Verification items for the finished model (mm, model axes). Round coordinates to 2 decimals unless told otherwise and drop trailing zeros. Order: outer loops, then holes, each group sorted by start corner. A loop starts at its lowest first (then second) coordinate and runs counter-clockwise, first axis right, second up. Notation, with made-up numbers: (-9, 3.25) -> (11, 3.25) arc R17 cw to (11, 25.25) -> close; hole circle Ø2 at (51, 74.5). An arc over 180 degrees is marked (long way). Write item = value, one per line. Start each with the question number.
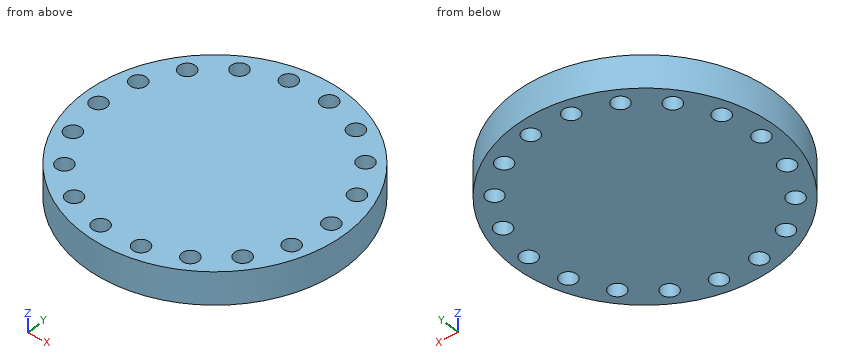
from build123d import *

# Parameters (mm, degrees)
SKETCH1_R           = 50.8
BOSS_EXTRUDE2_DEPTH = 12.7
SKETCH1_7_R         = 3.175
CUT_EXTRUDE1_DEPTH  = 12.7


with BuildPart() as part:
    # Sketch1 → Boss-Extrude2 (new body)
    with BuildSketch(Plane.XY):
        Circle(SKETCH1_R)
    extrude(amount=-BOSS_EXTRUDE2_DEPTH)

    # Sketch1<7> → Cut-Extrude1 (cut)
    with BuildSketch(Plane.XY):
        with Locations((-44.45, 0)):
            Circle(SKETCH1_7_R)
        with Locations((-41.769336994, 15.202795371)):
            Circle(SKETCH1_7_R)
        with Locations((-34.050675497, 28.571909251)):
            Circle(SKETCH1_7_R)
        with Locations((-22.225, 38.494829198)):
            Circle(SKETCH1_7_R)
        with Locations((-7.718661497, 43.774704621)):
            Circle(SKETCH1_7_R)
        with Locations((7.718661497, 43.774704621)):
            Circle(SKETCH1_7_R)
        with Locations((22.225, 38.494829198)):
            Circle(SKETCH1_7_R)
        with Locations((34.050675497, 28.571909251)):
            Circle(SKETCH1_7_R)
        with Locations((41.769336994, 15.202795371)):
            Circle(SKETCH1_7_R)
        with Locations((44.45, 0)):
            Circle(SKETCH1_7_R)
        with Locations((41.769336994, -15.202795371)):
            Circle(SKETCH1_7_R)
        with Locations((34.050675497, -28.571909251)):
            Circle(SKETCH1_7_R)
        with Locations((22.225, -38.494829198)):
            Circle(SKETCH1_7_R)
        with Locations((7.718661497, -43.774704621)):
            Circle(SKETCH1_7_R)
        with Locations((-7.718661497, -43.774704621)):
            Circle(SKETCH1_7_R)
        with Locations((-22.225, -38.494829198)):
            Circle(SKETCH1_7_R)
        with Locations((-34.050675497, -28.571909251)):
            Circle(SKETCH1_7_R)
        with Locations((-41.769336994, -15.202795371)):
            Circle(SKETCH1_7_R)
    extrude(amount=-CUT_EXTRUDE1_DEPTH, mode=Mode.SUBTRACT)


solid = part.part
(1) Cross-section at B-B (x = -35.5). Enter the section's corners in (y, z), and give its area (3 significant figures).
(2) Cross-section at D-D (y = 22). Enter the section's corners in (x, z).
(3) Depth check by flat-ended pin: pin 1 (4 mm diameter, centred on x = 34.05, y = 28.57, fed in from -Z); pin 2 (7.5 mm diameter, centred on x = 41.77, y = -15.2, fed in from -Z); pin 3 (3 mm diameter, centred on y = -4.5, z = -11.5, fed in from -X); pin 4 (5 mm diameter, centred on y = -3.5, z = -10.5, fed in from +X). Enter the tip coordinate at first touch or a pass-through.
(4) Scan lines: line 1 along X through (y, z) = (-31, -0.75); line 2 along X through (y, z) = (-40, -11); line 3 along Y through (x, z) = (-6.5, -4.5). Record each from-to range of solid material in increasing order. Write a range as from..to.
(5) Cross-section at C-C (z = -3.5). Give the number of separate pieces and of enclosed holes in the cut face, and give its area (3 significant figures).
(6) Cross-section at A-A (y = 0). Enter the section's corners in (x, z) (3 decimals), and give its area (3 significant figures).
Outcome:
q1.outline = (-36.34, -12.7) -> (-31.4, -12.7) -> (-31.4, 0) -> (-36.34, 0) -> close; (-25.75, -12.7) -> (25.75, -12.7) -> (25.75, 0) -> (-25.75, 0) -> close; (31.4, -12.7) -> (36.34, -12.7) -> (36.34, 0) -> (31.4, 0) -> close
q1.area = 779 mm^2
q2.outline = (-45.79, -12.7) -> (45.79, -12.7) -> (45.79, 0) -> (-45.79, 0) -> close
q3.pin_1 = through
q3.pin_2 = -12.7
q3.pin_3 = -50.71
q3.pin_4 = 50.79
q4.line_1 = -40.24..-36.1, -32..32, 36.1..40.24
q4.line_2 = -31.32..-25.02, -19.43..19.43, 25.02..31.32
q4.line_3 = -50.38..-46.71, -40.84..40.84, 46.71..50.38
q5.separate_pieces = 1
q5.enclosed_holes = 18
q5.area = 7,540 mm^2
q6.outline = (-50.8, -12.7) -> (-47.625, -12.7) -> (-47.625, 0) -> (-50.8, 0) -> close; (-41.275, -12.7) -> (41.275, -12.7) -> (41.275, 0) -> (-41.275, 0) -> close; (47.625, -12.7) -> (50.8, -12.7) -> (50.8, 0) -> (47.625, 0) -> close
q6.area = 1,130 mm^2
